Verification items for the finished model (mm, model axes). A direction names the side the tool comes from. Give positions to 0.01 mm unless a question says otherwise; leave off trailing zeros. Loops run counter-clockwise (first coordinate to the right, second up) from the corner with the lowest first, then second, coordinate; pieces in that order, holes last. Notation, with made-up numbers: (-21, 54) - (5, 54) arc R25 cw to (5, 92) - close; hole circle Ø4 at (-24, -25.75). An arc over 180 degrees is marked (long way). Put each result on its own line as item: value. Start each with the question number.
```python
from build123d import *

# Parameters (mm, degrees)
SKETCH_1_R             = 1.5
EXTRUDE_1_DEPTH        = 1.6
SKETCH_2_W             = 16.4
SKETCH_2_H             = 12.4
EXTRUDE_2_DEPTH        = 11.3
SKETCH_3_W             = 3
SKETCH_3_H             = 5.4
CUT_EXTRUDE_1_DEPTH    = 9
EXTRUDE_3_DEPTH        = 1.8
SKETCH_5_W             = 1
SKETCH_5_H             = 11
EXTRUDE_4_DEPTH        = 3
FILLET_1_R             = 0.5
SKETCH_43_W            = 8.3
SKETCH_43_H            = 52.3
EXTRUDE_15_DEPTH       = 7
SKETCH_45_W            = 6.9
SKETCH_45_H            = 38.3
CUT_EXTRUDE_12_DEPTH   = 6
SKETCH_53_W            = 16
SKETCH_53_H            = 12
EXTRUDE_20_DEPTH       = 12.2
SKETCH_54_W            = 6.55
SKETCH_54_H            = 12
CUT_EXTRUDE_14_DEPTH   = 5
SKETCH_59_R            = 1.6
CUT_EXTRUDE_16_DEPTH   = 10
PATTERN_LINEAR_4_COUNT = 2
PATTERN_LINEAR_4_PITCH = 22
SKETCH_60_W            = 5
SKETCH_60_H            = 5.8
EXTRUDE_21_DEPTH       = 3.15
SKETCH_61_W            = 2.1
SKETCH_61_H            = 0.78
EXTRUDE_22_DEPTH       = 8.2
SKETCH_62_W            = 0.6
SKETCH_62_H            = 0.835930121
EXTRUDE_23_DEPTH       = 6.9
EXTRUDE_23_DEPTH_BACK  = 6


with BuildPart() as part:
    # Sketch 1 → Extrude 1 (new body)
    with BuildSketch(Plane.XY):
        with BuildLine():
            Line((58, -60), (-58, -60))
            ThreePointArc((-58, -60), (-59.414213562, -59.414213562), (-60, -58))
            Line((-60, -58), (-60, 58))
            ThreePointArc((-60, 58), (-59.414213562, 59.414213562), (-58, 60))
            Line((-58, 60), (58, 60))
            ThreePointArc((58, 60), (59.414213562, 59.414213562), (60, 58))
            Line((60, 58), (60, -58))
            ThreePointArc((60, -58), (59.414213562, -59.414213562), (58, -60))
        make_face()
        with Locations((24, 55)):
            Circle(SKETCH_1_R, mode=Mode.SUBTRACT)
        with Locations((24, -56)):
            Circle(SKETCH_1_R, mode=Mode.SUBTRACT)
    extrude(amount=EXTRUDE_1_DEPTH)

    # Sketch 2 → Extrude 2 (add)
    with BuildSketch(Plane.XY.offset(1.6)):
        with Locations((-52.8, 28.9)):
            Rectangle(SKETCH_2_W, SKETCH_2_H)
    extrude(amount=EXTRUDE_2_DEPTH)

    # Sketch 3 → Cut-Extrude 1 (cut)
    with BuildSketch(Plane.ZY.offset(61)):
        Polygon((3, 33.7), (3, 24.1), (9.9, 24.1), (11.5, 25.7), (11.5, 32.1), (9.9, 33.7), align=None)
        with Locations((6.9, 28.9)):
            Rectangle(SKETCH_3_W, SKETCH_3_H, mode=Mode.SUBTRACT)
    extrude(amount=-CUT_EXTRUDE_1_DEPTH, mode=Mode.SUBTRACT)

    # Sketch 4 → Extrude 3 (add)
    with BuildSketch(Plane.XY.offset(1.6)):
        Polygon((-47.6, -18.8), (-47.6, -33.8), (-62.4, -33.8), (-62.4, -29.5), (-61.8, -23.188583942), (-61.8, -18.8), align=None)
    extrude(amount=EXTRUDE_3_DEPTH)

    # Sketch 5 → Extrude 4 (add)
    with BuildSketch(Plane.ZY.offset(61.8)):
        with Locations((2.8, -25.1)):
            Rectangle(SKETCH_5_W, SKETCH_5_H)
    extrude(amount=EXTRUDE_4_DEPTH)

    # Fillet 1
    fillet_1_edges = [part.edges().sort_by_distance(p)[0] for p in [
        (-64.8, -19.6, 2.8),
        (-64.8, -30.6, 2.8),
    ]]
    fillet(fillet_1_edges, radius=FILLET_1_R)

    # Sketch 43 → Extrude 15 (add)
    with BuildSketch(Plane(origin=(66.890855613, 85.562649537, 1.6), x_dir=(1, 0, 0), z_dir=(0, 0, 1))):
        with Locations((-11.040855613, -51.712649537)):
            Rectangle(SKETCH_43_W, SKETCH_43_H)
        with Locations((-11.040855613, -119.412649537)):
            Rectangle(SKETCH_43_W, SKETCH_43_H)
    extrude(amount=EXTRUDE_15_DEPTH)

    # Sketch 45 → Cut-Extrude 12 (cut)
    with BuildSketch(Plane(origin=(66.890855613, 85.562649537, 8.6), x_dir=(1, 0, 0), z_dir=(0, 0, 1))):
        with Locations((-11.040855613, -51.712649537)):
            Rectangle(SKETCH_45_W, SKETCH_45_H)
        with Locations((-11.040855613, -119.412649537)):
            Rectangle(SKETCH_45_W, SKETCH_45_H)
    extrude(amount=-CUT_EXTRUDE_12_DEPTH, mode=Mode.SUBTRACT)

    # Sketch 53 → Extrude 20 (add)
    with BuildSketch(Plane.XY.offset(1.6)):
        with Locations((-5.3, 54)):
            Rectangle(SKETCH_53_W, SKETCH_53_H)
    extrude_20 = extrude(amount=EXTRUDE_20_DEPTH)

    # Sketch 54 → Cut-Extrude 14 (cut)
    with BuildSketch(Plane.XY.offset(13.8)):
        with Locations((-9.225, 54)):
            Rectangle(SKETCH_54_W, SKETCH_54_H)
        with Locations((-1.375, 54)):
            Rectangle(SKETCH_54_W, SKETCH_54_H)
    cut_extrude_14 = extrude(amount=-CUT_EXTRUDE_14_DEPTH, mode=Mode.SUBTRACT)

    # Sketch 59 → Cut-Extrude 16 (cut)
    with BuildSketch(Plane.XY.offset(1.6)):
        with Locations((-40, -35)):
            Circle(SKETCH_59_R)
        with Locations((-40, 45)):
            Circle(SKETCH_59_R)
    extrude(amount=-CUT_EXTRUDE_16_DEPTH, mode=Mode.SUBTRACT)

    # Pattern Linear 4: Extrude 20, Cut-Extrude 14 ×2
    with Locations(*[(-i * PATTERN_LINEAR_4_PITCH, 0, 0) for i in range(1, PATTERN_LINEAR_4_COUNT)]):
        add(extrude_20)
        add(cut_extrude_14, mode=Mode.SUBTRACT)

    # Sketch 60 → Extrude 21 (add)
    with BuildSketch(Plane.XY.offset(1.6)):
        with Locations((-45.5, 57.1)):
            Rectangle(SKETCH_60_W, SKETCH_60_H)
    extrude(amount=EXTRUDE_21_DEPTH)

    # Sketch 61 → Extrude 22 (add)
    with BuildSketch(Plane.XY.offset(4.75)):
        with Locations((-45.5, 54.59)):
            Rectangle(SKETCH_61_W, SKETCH_61_H)
    extrude(amount=EXTRUDE_22_DEPTH)

    # Sketch 62 → Extrude 23 (add, two sides)
    with BuildSketch(Plane.XY.offset(4.75)) as extrude_23_sk:
        with Locations((-44.275, 57.657035773)):
            Rectangle(SKETCH_62_W, SKETCH_62_H)
        with Locations((-46.725, 57.657035773)):
            Rectangle(SKETCH_62_W, SKETCH_62_H)
    extrude(amount=EXTRUDE_23_DEPTH)
    extrude(extrude_23_sk.sketch, amount=-EXTRUDE_23_DEPTH_BACK)


solid = part.part
```
1) Section check A-A, the plane y = -56. Enter the section's corners in (x, z).
2) Section check B-B, the plane x = -40. Enter the section's corners in (y, z), plus the area to 3 significant figures.
3) Depth check by flat-ended pin: P1, Ø1, axis at y = 1, z = 3.5, coming from the +X side; P2, Ø10, axis at x = -55.5, y = 29, coming from the +Z side; P3, Ø1, axis at x = 59, y = -58.5, coming from the -Z side; P4, Ø3.5, axis at y = -26, z = 5.5, coming from the -X side. Enter the tip coordinate at first touch or a pass-through.
4) Section check C-C, the plane y = 45. Enter the section's corners in (x, z).
5) Draft check along X on faces 1 (the face through (-13.3, 54, 8)), 2 (the face through (56, 14.7, 6)), 3 (the face through (56, 7.7, 5)). Enter one of: pulls with the +X half, pulls with the -X half, needs draft (parallel to the pull), parting line crosses it, or undercut.
6) Section check D-D, the plane x = -8. Enter the section's corners in (y, z), plus the area to 3 significant figures.
7) Scan lines: line 1 along Y through (x, z) = (-40, 1.1); line 2 along X through (y, z) = (50, 11.25); line 3 along X through (y, z) = (33.5, 7.5). Record each from-to range of solid material in increasing order. Write a range as from..to.
8) Set-up check for faces 4 (the face through (-57, 33.7, 6)), 5 (the face through (1.9, 54, 11)), 6 (the face through (-55, -26, 3.4)), 7 (the face through (-44.6, 29, 7)), 8 (the face through (59.3, -34, 6)): record each of +Z, -Z, +X, -X, +Y, -Y from which the full face is reachable in a straight line by a thin tool's end or side.
Results are:
1. outline: (-60, 0) - (22.5, 0) - (22.5, 1.6) - (-60, 1.6) - close; (25.5, 0) - (60, 0) - (60, 8.6) - (51.7, 8.6) - (51.7, 1.6) - (25.5, 1.6) - close
2. outline: (-60, 0) - (-36.6, 0) - (-36.6, 1.6) - (-60, 1.6) - close; (-33.4, 0) - (43.4, 0) - (43.4, 1.6) - (-33.4, 1.6) - close; (46.6, 0) - (60, 0) - (60, 1.6) - (46.6, 1.6) - close
2. area: 182 mm2
3. P1: passes through
3. P2: stops at z = 12.9
3. P3: stops at z = 0
3. P4: stops at x = 51.7
4. outline: (-60, 0) - (-41.6, 0) - (-41.6, 1.6) - (-60, 1.6) - close; (-38.4, 0) - (60, 0) - (60, 8.6) - (59.3, 8.6) - (59.3, 2.6) - (52.4, 2.6) - (52.4, 8.6) - (51.7, 8.6) - (51.7, 1.6) - (-38.4, 1.6) - close
5. face 1: undercut
5. face 2: undercut
5. face 3: needs draft
6. outline: (-60, 0) - (60, 0) - (60, 8.8) - (48, 8.8) - (48, 1.6) - (-60, 1.6) - close
6. area: 278 mm2
7. line 1: y = -60..-36.6, -33.4..43.4, 46.6..60
7. line 2: x = -35.3..-34.5, -27.95..-26.65, -20.1..-19.3, -13.3..-12.5, -5.95..-4.65, 1.9..2.7
7. line 3: x = -52..-44.6, 51.7..52.4, 59.3..60
8. face 4: -X
8. face 5: +Z, +Y, -Y
8. face 6: +Z, -X, -Y
8. face 7: +Z, -Y
8. face 8: +Z
